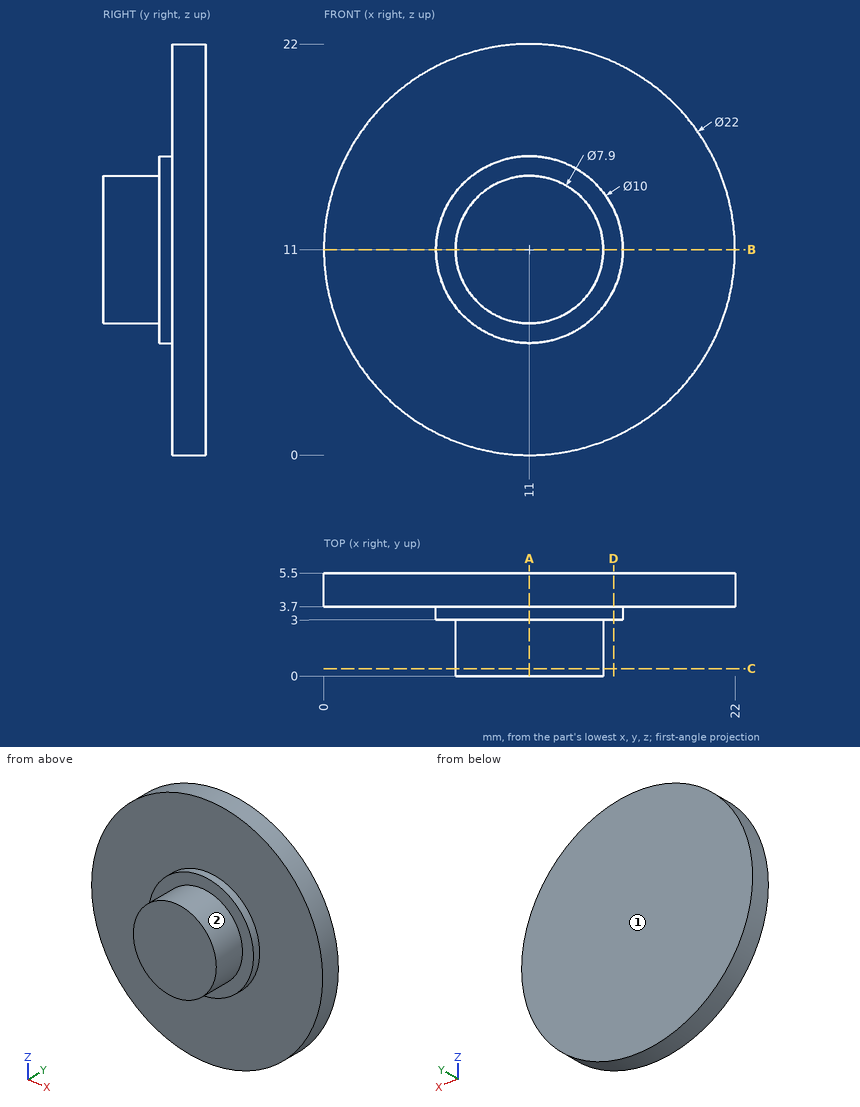
Job drawing, mm, ordinate dimensions from the low corner. One solid piece. A direction names the side the tool comes from. Round coordinates to 2 decimals unless told otherwise and drop trailing zeros. Write each loop counter-clockwise with the first axis right and the second up, starting at its lowest first coordinate (ties: lowest second). Pieces come first, ordered by that corner, then holes. Notation, with made-up numbers: M 80.25,36.25 L 108.25,36.25 A33 cw 108.25,70.25 Z; hole C -15.5,-19 d4. An arc over 180 degrees is marked long. Return JSON: item names as keys, results as strings. Group by question number.
(1) Which spindle directions (+Z, -Z, +X, -X, +Y, -Y) get a long thin tool onto all of the face, cutting with end or side? Do the marked faces 1 and 2. Say none if no direction does.
(2) Saw through at A-A on x = 11. Write the cut outline in (y, z).
(3) Saw through at C-C on y = 0.4. Write the cut outline in (x, z).
(4) Drill centre lines: probe 1 along Y at (x, z) = (8.5, 17.5); probe 2 along X at (y, z) = (4.15, 14); probe 3 along X at (y, z) = (4.6, 1). Where is each one in solid material? Low to high.
(5) Saw through at D-D on x = 15.5. Write the cut outline in (y, z).
(6) Saw through at B-B on z = 11. Write the cut outline in (x, y).
(7) Pin check, flat tips, straight feed: pin 1 Ø1.5 at (x, z) = (19.5, 12.5) entering from -Y; pin 2 Ø3 at (x, y) = (19, 3) entering from -Z; pin 3 Ø2 at (x, y) = (14.5, 1) entering from +Z. Stop position of each tip, or through.
Returned:
{
 "1": {"face 1": "+Z, -Z, +X, -X, +Y", "face 2": "-Y"},
 "2": {"outline": "M 0,7.05 L 3,7.05 L 3,6 L 3.7,6 L 3.7,0 L 5.5,0 L 5.5,22 L 3.7,22 L 3.7,16 L 3,16 L 3,14.95 L 0,14.95 Z"},
 "3": {"outline": "C 11,11 d7.9"},
 "4": {"probe 1": "3.7 to 5.5", "probe 2": "0.42 to 21.58", "probe 3": "6.42 to 15.58"},
 "5": {"outline": "M 3,8.82 L 3.7,8.82 L 3.7,0.96 L 5.5,0.96 L 5.5,21.04 L 3.7,21.04 L 3.7,13.18 L 3,13.18 Z"},
 "6": {"outline": "M 0,3.7 L 6,3.7 L 6,3 L 7.05,3 L 7.05,0 L 14.95,0 L 14.95,3 L 16,3 L 16,3.7 L 22,3.7 L 22,5.5 L 0,5.5 Z"},
 "7": {"pin 1": "y = 3.7", "pin 2": "z = 2.26", "pin 3": "z = 14.06"}
}
